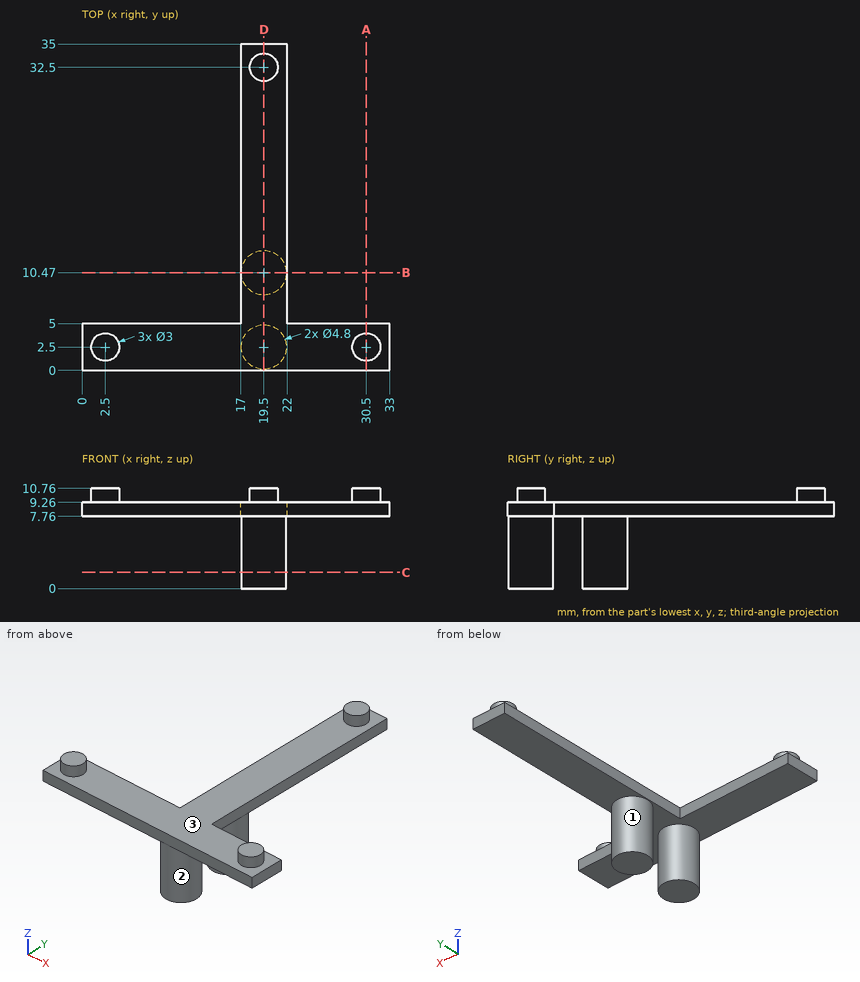
Design review of the part shown in the three views and the two pictorial views. Dimensions are in mm from the part's minimum x, y and z. Give positions to 0.01 mm unless a question says otherwise; leave off trailing zeros. Loops run counter-clockwise (first coordinate to the right, second up) from the corner with the lowest first, then second, coordinate; pieces in that order, holes last. Notation, with made-up numbers: (69, 25) - (85, 25) arc R20 cw to (85, 32) - close; hole circle Ø7 at (46, 44.5). An arc over 180 degrees is marked (long way). Write item = value, one per line.
1) Take a section at B-B on y = 10.47. State the section outline as (x, z) points.
Result sheet:
outline = (17, 7.76) - (17.1, 7.76) - (17.1, 0) - (21.9, 0) - (21.9, 7.76) - (22, 7.76) - (22, 9.26) - (17, 9.26) - close
2) Take a section at C-C on z = 1.75. State the section outline as (x, y) points, and give its area (3 significant figures).
Result sheet:
outline = circle Ø4.8 at (19.5, 2.5); circle Ø4.8 at (19.5, 10.47)
area = 36.2 mm2
3) Draft analysis for pull direction Y (two halves, no side actions). For the marked faces 1, 2 and 3, state which applies: +Y half, -Y half, draft (parallel to the pull), parting line (faces both ways), or undercut.
Result sheet:
face_1 = undercut
face_2 = undercut
face_3 = draft
4) Take a section at D-D on x = 19.5. State the section outline as (y, z) points, and give its area (3 significant figures).
Result sheet:
outline = (0, 7.76) - (0.1, 7.76) - (0.1, 0) - (4.9, 0) - (4.9, 7.76) - (8.07, 7.76) - (8.07, 0) - (12.87, 0) - (12.87, 7.76) - (35, 7.76) - (35, 9.26) - (34, 9.26) - (34, 10.76) - (31, 10.76) - (31, 9.26) - (0, 9.26) - close
area = 131 mm2
5) Take a section at A-A on x = 30.5. State the section outline as (y, z) points.
Result sheet:
outline = (0, 7.76) - (5, 7.76) - (5, 9.26) - (4, 9.26) - (4, 10.76) - (1, 10.76) - (1, 9.26) - (0, 9.26) - close
6) To check wall thickness, follow line 1 (Y direction, x = 19.5, z = 0.5); line 2 (Y direction, x = 30.5, z = 9.75); line 3 (X direction, y = 21.5, z = 8.25). State the ranges of each line that lie inside material, in increasing order.
Result sheet:
line_1 = 0.1 to 4.9, 8.07 to 12.87
line_2 = 1 to 4
line_3 = 17 to 22
7) Clearance check with flat-ended pins moving along their axes: pin 1 Ø1 at (x, z) = (26, 8.5) entering from +Y; pin 2 Ø2 at (y, z) = (15.5, 5) entering from -X; pin 3 Ø2 at (x, y) = (17.5, 24) entering from +Z. State where each tip first meets the part, or that it passes through.
Result sheet:
pin_1 = 5
pin_2 = through
pin_3 = 9.26
